For this review, take the finished solid that the model builds, in its own axes (mm). A direction names the side the tool comes from. Give positions to 0.01 mm unless a question says otherwise; leave off trailing zeros. Loops run counter-clockwise (first coordinate to the right, second up) from the corner with the lowest first, then second, coordinate; pieces in that order, holes last. Notation, with made-up numbers: (24, -12.75) - (55, -12.75) arc R19 ccw to (55, 10.25) - close; hole circle Ø5 at (25.5, 63). An arc over 180 degrees is marked (long way). Put each result on its own line as item: value.
from build123d import *

# Parameters (mm, degrees)
F0_R     = 12.7
F1_DEPTH = 38.862
F2_R     = 12.7
F2_R_2   = 7.3787
F3_DEPTH = 13.97
F5_DEPTH = 24.892
F6_W     = 1.03275
F6_H     = 24.892
F6_R     = 4.064
F7_DEPTH = 25.4


with BuildPart() as f1:
    # F0 (on Front) → F1 (new body)
    with BuildSketch(Plane.XZ):
        Circle(F0_R)
    extrude(amount=F1_DEPTH)

    # F2 (on face) → F3 (cut)
    with BuildSketch(Plane.XZ.offset(38.862)):
        Circle(F2_R)
        Circle(F2_R_2, mode=Mode.SUBTRACT)
    extrude(amount=-F3_DEPTH, mode=Mode.SUBTRACT)

    # F4 (on face) → F5 (cut)
    with BuildSketch(Plane(origin=(0, 0, 0), x_dir=(-1, 0, 0), z_dir=(0, 1, 0))):
        with BuildLine():
            ThreePointArc((11.66725, 5.0165), (0, 12.7), (-11.66725, 5.0165))
            Line((-11.66725, 5.0165), (11.66725, 5.0165))
        make_face()
        with BuildLine():
            Line((11.66725, -5.0165), (-11.66725, -5.0165))
            ThreePointArc((-11.66725, -5.0165), (0, -12.7), (11.66725, -5.0165))
        make_face()
    extrude(amount=-F5_DEPTH, mode=Mode.SUBTRACT)

    # F6 (on face) → F7 (cut)
    with BuildSketch(Plane.XY.offset(5.0165)):
        with BuildLine():
            Line((-11.66725, 0), (-11.66725, -24.892))
            Line((-11.66725, -24.892), (-7.3787, -24.892))
            Line((-7.3787, -24.892), (-10.291934, -13.160184))
            ThreePointArc((-10.291934, -13.160184), (-8.353358, -4.071749), (0, 0))
            Line((0, 0), (-11.66725, 0))
        make_face()
        with Locations((-12.183625, -12.446)):
            Rectangle(F6_W, F6_H)
        with BuildLine():
            Line((11.66725, 0), (0, 0))
            ThreePointArc((0, 0), (7.498514, -3.105986), (10.6045, -10.6045))
            ThreePointArc((10.6045, -10.6045), (10.526068, -11.891863), (10.291934, -13.160184))
            Line((10.291934, -13.160184), (7.3787, -24.892))
            Line((7.3787, -24.892), (11.66725, -24.892))
            Line((11.66725, -24.892), (11.66725, 0))
        make_face()
        with Locations((12.183625, -12.446)):
            Rectangle(F6_W, F6_H)
        with Locations((0, -10.3886)):
            Circle(F6_R)
    extrude(amount=-F7_DEPTH, mode=Mode.SUBTRACT)


solid = f1.part
1) Take a section at B-B on x = -0.5. State the section outline as (y, z) points, and give its area (3 significant figures).
Geometry check:
outline: (-38.86, -7.36) - (-24.89, -7.36) - (-24.89, -5.02) - (-14.42, -5.02) - (-14.42, 5.02) - (-24.89, 5.02) - (-24.89, 7.36) - (-38.86, 7.36) - close; (-6.36, -5.02) - (-0.01, -5.02) - (-0.01, 5.02) - (-6.36, 5.02) - close
area: 374 mm²
2) Take a section at C-C on y = -32.5. State the section outline as (x, z) points.
Geometry check:
outline: circle Ø14.76 at (0, 0)
3) Draft analysis for pull direction X (two halves, no side actions). For faces 1 (the face through (7.038, -31.975, 2.216)), 2 (the face through (8.856, -18.944, 0.07)), 3 (the face through (-0.53, -6.36, 0.07)), state which applies: pulls with the +X half, pulls with the -X half, needs draft (parallel to the pull), parting line crosses it, or undercut.
Geometry check:
face 1: parting line crosses it
face 2: pulls with the +X half
face 3: undercut
4) Take a section at D-D on x = 5. State the section outline as (y, z) points, and give its area (3 significant figures).
Geometry check:
outline: (-38.86, -5.43) - (-24.89, -5.43) - (-24.89, -5.02) - (-1.25, -5.02) - (-1.25, 5.02) - (-24.89, 5.02) - (-24.89, 5.43) - (-38.86, 5.43) - close
area: 389 mm²
5) Wall thickness on line 1 (Y direction, x = 0, z = -1.5); line 2 (Z direction, x = -9, y = -17); line 3 (X direction, y = -11, z = 2.5): over which ranges is each line inside the solid? List them lowest first.
Geometry check:
line 1: y = -38.86 to -14.45, -6.32 to 0
line 2: z = -5.02 to 5.02
line 3: x = -10.6 to -4.02, 4.02 to 10.6
6) Take a section at A-A on z = -4.25. State the section outline as (x, y) points.
Geometry check:
outline: (-10.29, -13.16) - (-7.38, -24.89) - (-6.03, -24.89) - (-6.03, -38.86) - (6.03, -38.86) - (6.03, -24.89) - (7.38, -24.89) - (10.29, -13.16) arc R10.6 ccw to (10.6, -10.6) arc R10.6 ccw (long way) to start; hole circle Ø8.13 at (0, -10.39)
7) For faces 4 (the face through (-7, -24.892, 4)), 5 (the face through (0, -24.892, 6)), 6 (the face through (0, -24.892, -6)), list the 3-axis set-ups (+Z, -Z, +X, -X, +Y, -Y) from which the entire face can be reached by the end or side of a thin tool; tool diameter is ignored.
Geometry check:
face 4: +Z, -X, -Y
face 5: +Z, +X, -X, +Y
face 6: -Z, +X, -X, +Y
8) Insertion check: pin 1 Ø5 at (x, y) = (-2, -20) entering from +Z; pin 2 Ø3 at (y, z) = (-6.5, -6) entering from -X; pin 3 Ø1.2 at (x, z) = (-0.5, 6) entering from +Y. Each pin has a flat end and moves straight along its axis. Give the tip position at first contact, or say it passes through.
Geometry check:
pin 1: stops at z = 5.02
pin 2: stops at x = -10.18
pin 3: stops at y = -24.89
